Could you check a few things on this model? Use its own coordinates, in mm. A direction names the side the tool comes from. Coordinates: 2 decimals unless noted, no trailing zeros. Loops run counter-clockwise (first coordinate to the right, second up) from the corner with the lowest first, then second, coordinate; pieces in that order, holes last.
1) Thinking about a two-plate mould opening in Z: for faces 6 (the face through (-5, 0, 4)), 7 (the face through (-0.43, 35.55, 56.5)), 8 (the face through (8, 36, 1.5)), which applies, released by +Z, released by -Z, zero draft, split by the parting line, or undercut?
2) Imagine slicing it at A-A on y = 60. Please give me the cut outline in (x, z).
3) For faces 1 (the face through (-6.24, 18.38, 15.57)), 2 (the face through (-2.5, 28, 8)), 3 (the face through (1, 36.252, 18)), 4 (the face through (-18, 68, 34)), 5 (the face through (-12.77, 36.45, 46)), which set-ups out of +Z, -Z, +X, -X, +Y, -Y let a thin tool reach every point of the face, with its end or its side?
4) Imagine slicing it at C-C on x = -31.5. Please give me the cut outline in (y, z), plus the area to 3 significant figures.
5) Imagine slicing it at D-D on y = 41. Please give me the cut outline in (x, z), plus the area to 3 significant figures.
6) If I drill on line 1 along X through (y, z) = (24, 13.5); line 2 along Z through (x, y) = (-31, 27.5); line 3 along Z through (x, y) = (-2.5, 9), over which ranges is the centre line in solid material (lowest first)?
7) Will these pins go through, and if not, where does the flat tip stop? P1, Ø4, axis at y = 44.5, z = 47.5, coming from the -X side; P2, Ø12, axis at x = -15, z = 18, coming from the +Y side; P3, Ø24, axis at y = 28.5, z = 19, coming from the +X side; P4, Ø10, axis at x = -11.5, z = 30.5, coming from the +Y side.
8) Imagine slicing it at B-B on z = 28. Please give me the cut outline in (x, y), plus the area to 3 significant figures.
```python
from build123d import *

# Parameters (mm, degrees)
F3_W     = 5
F3_H     = 20
F3_R     = 40
F5_DEPTH = 1.5
F6_W     = 3
F6_H     = 64


with BuildPart() as f2:
    # F2: sweep along a path in F1
    with BuildLine(Plane.YZ) as f2_path:
        Line((0, 0), (36.2523114815, 16.9047304696))
    # F0 (on Front) → F2 (sweep)
    with BuildSketch(Plane.XZ):
        with BuildLine():
            Line((-5.5, 7), (-7, 7))
            ThreePointArc((-7, 7), (0, 0), (7, 7))
            Line((7, 7), (5.5, 7))
            ThreePointArc((5.5, 7), (0, 1.5), (-5.5, 7))
        make_face()
    sweep(path=f2_path.line)

    # F3 (on Top) → F4 (join, up to the next surface of F2)
    with BuildSketch(Plane.XY):
        with Locations((0, 26)):
            Rectangle(F3_W, F3_H)
    extrude(until=Until.NEXT)

    # F3 (on Top) → F5 (join)
    with BuildSketch(Plane.XY):
        with Locations((0, 35)):
            Circle(F3_R)
        with Locations((0, 26)):
            Rectangle(F3_W, F3_H, mode=Mode.SUBTRACT)
    extrude(amount=F5_DEPTH)

    # F9: sweep along a path in F8
    with BuildLine(Plane.XZ.offset(-68)) as f9_path:
        Line((-17.4873532057, 1.5), (-17.4873532057, 31.5))
        ThreePointArc((-17.4873532057, 31.5), (-12.6384664104, 46.1788768101), (0, 55.08114025))
    # F6 (on face) → F9 (sweep)
    with BuildSketch(Plane.XY.offset(1.5)):
        with Locations((-18.9873532057, 36)):
            Rectangle(F6_W, F6_H)
    sweep(path=f9_path.line)


solid = f2.part
```
Filled in:
1. face 6: zero draft
1. face 7: released by +Z
1. face 8: undercut
2. outline: (-31.22, 0) - (31.22, 0) - (31.22, 1.5) - (-17.49, 1.5) - (-17.49, 31.5) arc R24.64 cw to (0, 55.08) - (-0.87, 57.95) arc R27.64 ccw to (-20.49, 31.5) - (-20.49, 1.5) - (-31.22, 1.5) - close
3. face 1: +X, -Y
3. face 2: +Y
3. face 3: +X, +Y
3. face 4: +Z, +X, -X, +Y
3. face 5: +X, +Y, -Y
4. outline: (10.35, 0) - (59.65, 0) - (59.65, 1.5) - (10.35, 1.5) - close
4. area: 74.0 mm2
5. outline: (-39.55, 0) - (39.55, 0) - (39.55, 1.5) - (-17.49, 1.5) - (-17.49, 31.5) arc R24.64 cw to (0, 55.08) - (-0.87, 57.95) arc R27.64 ccw to (-20.49, 31.5) - (-20.49, 1.5) - (-39.55, 1.5) - close
5. area: 309 mm2
6. line 1: x = -20.49 to -17.49, -5.2 to -2.87, 2.87 to 5.2
6. line 2: z = 0 to 1.5
6. line 3: z = 0 to 1.5, 4.66 to 6.3, 54.17 to 57.4
7. P1: stops at x = -16.68
7. P2: stops at y = 68
7. P3: stops at x = 7
7. P4: passes through
8. outline: (-20.49, 4) - (-17.49, 4) - (-17.49, 68) - (-20.49, 68) - close
8. area: 192 mm2
